from build123d import *

# Parameters (mm, degrees)
F1_DEPTH = 18


# Not quite as in the source:
# - a feature of the source that left no trace in its solid (it failed there, or was rolled back) is left out


with BuildPart() as f1:
    # F0 (on Front) → F1 (new body)
    with BuildSketch(Plane.XZ):
        with BuildLine():
            Line((295, -217), (-326, -217))
            add(Edge.make_bspline(
                [(0, -626), (-31.9041572511, -632.8686919212), (-135.8624745728, -641.8458876021), (-249.8265846826, -605.2490014373), (-303.9460461433, -495.6098595325), (-325.4699671722, -417.4111427766), (-326, -217)],
                knots=[0, 0, 0, 0, 0.234743673, 0.4538776177, 0.6453771431, 1, 1, 1, 1], degree=3))
            Line((0, -626), (0, -329))
            Line((0, -329), (295, -329))
            Line((295, -329), (295, -217))
        make_face()
        with BuildLine():
            add(Edge.make_bspline(
                [(0, 192), (-31.9041572511, 198.8686919212), (-135.8624745728, 207.8458876021), (-249.8265846826, 171.2490014373), (-303.9460461433, 61.6098595325), (-325.4699671722, -16.5888572234), (-326, -217)],
                knots=[0, 0, 0, 0, 0.234743673, 0.4538776177, 0.6453771431, 1, 1, 1, 1], degree=3))
            Line((-326, -217), (295, -217))
            Line((295, -217), (295, -105))
            Line((295, -105), (0, -105))
            Line((0, -105), (0, 192))
        make_face()
    extrude(amount=F1_DEPTH)


solid = f1.part
Input: part model. Units: mm. Frame: model coordinates. A direction names the side the tool comes from. Coordinates: 2 decimals unless noted, no trailing zeros. Order: outer loops, then holes, each group sorted by start corner. A loop starts at its lowest first (then second) coordinate and runs counter-clockwise, first axis right, second up. Notation, with made-up numbers: M -15,52.5 L -5,52.5 A27 cw -5,86.5 Z; hole C 1,72 d2. An arc over 180 degrees is marked long. Answer as CSV lines item,"result".
1. Access query for faces 1 (the flat face through (295, -9, -219)), 2 (the flat face through (0, -9, 41)), 3 (the flat face through (145, -9, -329)). Directions: +Z, -Z, +X, -X, +Y, -Y. A direction counts if a zero-diameter tool reaches every point of the face in a straight line with its end or side. Return the directions, or none.
Reported:
face 1,"+Z, -Z, +X, +Y, -Y"
face 2,"+Z, +X, +Y, -Y"
face 3,"-Z, +X, +Y, -Y"
2. Material intervals for line 1 (Z direction, x = 264.5, y = -6.75); line 2 (X direction, y = -3.5, z = -216.5); line 3 (X direction, y = -8.5, z = -4.5), sorted ascending. Write a range as from..to.
Reported:
line 1,"-329..-105"
line 2,"-326..295"
line 3,"-315.11..0"
3. Section A-A (x = 32). Return the cut outline in (y, z), then the cut area to 3 significant figures.
Reported:
outline,"M -18,-329 L 0,-329 L 0,-105 L -18,-105 Z"
area,"4,030 mm2"
4. First-contact query: P1, Ø9, axis at x = 168, y = -5, coming from the -Z side; P2, Ø5.5, axis at y = -12, z = 97.5, coming from the +X side; P3, Ø3, axis at y = -6, z = -412.5, coming from the -X side. Flat tips, straight axial feed; report the tip coordinate or a pass-through.
Reported:
P1,"z = -329"
P2,"x = 0"
P3,"x = -317.6"
